Verification items for the finished model (mm, model axes). A direction names the side the tool comes from. Round coordinates to 2 decimals unless told otherwise and drop trailing zeros. Write each loop counter-clockwise with the first axis right and the second up, starting at its lowest first coordinate (ties: lowest second). Pieces come first, ordered by that corner, then holes. Notation, with made-up numbers: M -28,-27 L 9,-27 A15 cw 9,-20 Z; hole C -36.5,63.25 d5. An arc over 180 degrees is marked long. One line per item, written item: value. Start each with the question number.
Item 1: Draft check along X on faces 1 (the face through (0.37, -22.54, 29.85)), 2 (the face through (22.226, -52, 3)), 3 (the face through (-0.311, -52.365, 33.735)). Enter one of: +X half, -X half, draft (parallel to the pull), parting line (faces both ways), or undercut.
Item 2: Section check A-A, the plane x = -44.45. Record the cut outline in (y, z), then the cut area to 3 significant figures.
Item 3: Tool access check on faces 4 (the face through (-57.15, -3, 1)), 5 (the face through (-22.226, -52, 3)), 6 (the face through (24.56, -22.54, -0.44)), 7 (the face through (45, -6.35, 1)), 8 (the face through (0, -52, -27.515)). Record the directions out of +Z, -Z, +X, -X, +Y, -Y that give a thin tool (end or side, any length) a straight path to the whole face; none if there is none.
Item 4: Section check B-B, the plane x = 46. Record the cut outline in (y, z).
Item 5: Gauge pin test, flat ends, axial feed: pin 1 (1.6 mm diameter, centred on y = -52.5, z = 17, fed in from -X); pin 2 (3.5 mm diameter, centred on x = -6.5, y = -52, fed in from -Z); pin 3 (6 mm diameter, centred on y = -23, z = 10, fed in from +X). Record the tip position at first contact, or that the pin passes through.
Item 6: Thickness scan on probe 1 along Z at (x, y) = (0, -50.5); probe 2 along X at (y, z) = (-5, 13); probe 3 along Y at (x, z) = (3, 2) (3 decimals). Record the ranges inside material, lowest first. Write a range as from..to.
from build123d import *

# Parameters (mm, degrees)
F0_W      = 65.620646
F0_H      = 76.2
F1_DEPTH  = 50.8
F1_TAPER  = 4.765
F2_T      = -6.35
F3_W      = 44.4515540981
F3_H      = 61.380908036
F4_DEPTH  = 3.175
F5_W      = 52.8765998903
F5_H      = 63.4559538903
F6_DEPTH  = 6.35
F7_R      = 127
F8_DEPTH  = 4.4846550372
F9_R      = 114.3
F10_DEPTH = 4.4846550455
F11_R     = 3.96875
F12_DEPTH = 53.9760001
F13_R     = 4.7625
F14_DEPTH = 53.9760001


with BuildPart() as f1:
    # F0 (on Front) → F1 (new body)
    with BuildSketch(Plane.XZ):
        Rectangle(F0_W, F0_H)
    extrude(amount=F1_DEPTH, taper=F1_TAPER)

    # F2
    f2_openings = [f1.faces().sort_by_distance(p)[0] for p in [
        (0, 0, 0),
    ]]
    offset(amount=F2_T, openings=f2_openings)

    # F3 (on face) → F4 (join)
    with BuildSketch(Plane.XZ.offset(50.8)):
        with Locations((0, 3.174999969)):
            Rectangle(F3_W, F3_H)
    extrude(amount=F4_DEPTH)

    # F5 (on Front) → F6 (join)
    with BuildSketch(Plane.XZ):
        Polygon((-32.810323, -38.1), (32.810323, -38.1), (57.15, -38.1), (57.15, 38.1), (32.810323, 38.1), (-32.810323, 38.1), (-57.15, 38.1), (-57.15, -38.1), align=None)
        Rectangle(F5_W, F5_H, mode=Mode.SUBTRACT)
    extrude(amount=F6_DEPTH)

    # F7 (on face) → F8 (cut, through all)
    with BuildSketch(Plane(origin=(0, -3.1539942218, 37.8370918571), x_dir=(1, 0, 0), z_dir=(0, -0.0830691049, 0.9965437892))):
        with Locations((28.5757769869, -47.8112515417)):
            Circle(F7_R)
    extrude(amount=F8_DEPTH, mode=Mode.SUBTRACT)

    # F9 (on face) → F10 (cut, through all)
    with BuildSketch(Plane(origin=(0, -3.1539942218, -37.8370918571), x_dir=(1, 0, 0), z_dir=(0, -0.0830691049, -0.9965437892))):
        with Locations((-28.5757769869, 47.8112515417)):
            Circle(F9_R)
    extrude(amount=F10_DEPTH, mode=Mode.SUBTRACT)

    # F11 (on face) → F12 (cut, through all)
    with BuildSketch(Plane(origin=(0, 0, 0), x_dir=(-1, 0, 0), z_dir=(0, 1, 0))):
        with Locations((-44.45, 12.7)):
            Circle(F11_R)
        with Locations((44.45, 12.7)):
            Circle(F11_R)
    extrude(amount=-F12_DEPTH, mode=Mode.SUBTRACT)

    # F13 (on face) → F14 (cut, through all)
    with BuildSketch(Plane.XZ.offset(53.975)):
        with Locations((0, 7.4095460131)):
            Circle(F13_R)
    extrude(amount=-F14_DEPTH, mode=Mode.SUBTRACT)


solid = f1.part
Response values:
1. face 1: undercut
1. face 2: +X half
1. face 3: draft
2. outline: M -6.35,-37.57 L 0,-38.1 L 0,8.73 L -6.35,8.73 Z; M -6.35,16.67 L 0,16.67 L 0,38.1 L -6.35,37.57 Z
2. area: 430 mm2
3. face 4: +Z, -Z, -X, +Y, -Y
3. face 5: +Z, -Z, -X, -Y
3. face 6: +Y
3. face 7: +Z, -Z, +X, -Y
3. face 8: -Z, +X, -X, -Y
4. outline: M -6.35,-37.57 L 0,-38.1 L 0,9.05 L -6.35,9.05 Z; M -6.35,16.35 L 0,16.35 L 0,38.1 L -6.35,37.57 Z
5. pin 1: stops at x = -22.23
5. pin 2: stops at z = -33.91
5. pin 3: stops at x = 31.14
6. probe 1: z = -33.89..2.65, 12.17..33.89
6. probe 2: x = -57.15..-48.41, -40.49..-26.02, 26.02..40.49, 48.41..57.15
6. probe 3: y = -53.975..-44.45
